Autodesk Inventor part; units mm, degrees
ref_plane "YZ Plane" through (0, 0, 0) normal (1, 0, 0) x (0, 1, 0)
ref_plane "XZ Plane" through (0, 0, 0) normal (0, 1, 0) x (-1, 0, 0)
ref_plane "XY Plane" through (0, 0, 0) normal (0, 0, 1) x (1, 0, 0)
sketch "Boceto1" plane through (0, 0, 0) normal (0, 0, 1) x (1, 0, 0)
  line L0 (-71.1055, 70.4875) -> (71.7516, 70.4875) construction
  line L1 (71.7516, 70.4875) -> (71.7516, -69.9887) construction
  line L2 (71.7516, -69.9887) -> (-71.1055, -69.9887) construction
  line L3 (-71.1055, -69.9887) -> (-71.1055, 70.4875) construction
  line L4 (-16.344, -18.0372) -> (15.0954, -18.0372)
  point P0 (0, 0)
sketch "Boceto2" plane through (0, 0, 0) normal (0, 0, 1) x (1, 0, 0)
  line L0 (-30.1866, -53.4632) -> (28.6068, -53.4632)
  line L1 (28.6068, -53.4632) -> (28.6068, -45.7841)
  line L2 (28.6068, -45.7841) -> (25.4871, -40.2647)
  line L3 (25.4871, -40.2647) -> (25.4871, -33.3055)
  line L4 (25.4871, -33.3055) -> (19.4878, -25.8663)
  line L5 (19.4878, -25.8663) -> (17.4099, -23.2897)
  line L6 (17.4099, -23.2897) -> (17.4099, -19.147)
  line L7 (17.4099, -19.147) -> (15.8731, -17.2414)
  line L8 (15.8731, -17.2414) -> (15.8731, -13.8176)
  line L9 (15.8731, -13.8176) -> (28.6068, -13.8176)
  line L10 (28.6068, -13.8176) -> (28.6068, 15.1601)
  line L11 (-30.1866, -53.4632) -> (-30.1866, -45.7841)
  line L12 (-30.1866, -45.7841) -> (-26.4512, -40.2647)
  line L13 (-26.4512, -40.2647) -> (-27.2401, -37.2121)
  line L14 (-27.2401, -37.2121) -> (-27.2401, -33.9857)
  line L15 (-27.2401, -33.9857) -> (-19.5651, -22.6451)
  line L16 (-19.5651, -22.6451) -> (-19.5651, -19.9512)
  line L17 (-19.5651, -19.9512) -> (-16.9146, -18.1942)
  line L18 (-16.9146, -18.1942) -> (-16.9146, -13.8176)
  line L19 (-16.9146, -13.8176) -> (-24.4978, -13.8176)
  arc A0 (-6.2899, 13.0619) -> (-24.4978, -13.8176) centre (7.8446, -16.1193) ccw
  arc A1 (-6.2899, 13.0619) -> (-2.4548, 26.1011) centre (-14.9411, 22.69) ccw
  line L20 (-2.4548, 26.1011) -> (-10.0959, 22.69)
  line L21 (-10.0959, 22.69) -> (-13.96, 24.3955)
  line L22 (-13.96, 24.3955) -> (-25.9619, 19.0376)
  arc A2 (-30.1866, 30.1701) -> (-25.9619, 19.0376) centre (-21.015, 27.2828) ccw
  line L23 (-30.1866, 30.1701) -> (-19.0004, 38.444)
  line L24 (-19.0004, 38.444) -> (-15.9019, 45.9592)
  line L25 (-15.9019, 45.9592) -> (-7.7883, 50.5452)
  line L26 (-7.7883, 50.5452) -> (-10.0959, 56.9512)
  arc A3 (2.199, 50.5452) -> (-10.0959, 56.9512) centre (-7.6346, 46.6736) ccw
  arc A4 (28.6068, 20.3485) -> (2.199, 50.5452) centre (-1.5881, 20.5877) ccw
  line L27 (28.6068, 20.3485) -> (28.6068, -13.8176)
  line L28 (-16.9146, -13.8176) -> (15.8731, -13.8176)
  point P0 (0, 0)
extrude "Extrusión1" add sketch "Boceto2" along normal blind 10
sketch "Boceto3" plane through (0, 0, 10) normal (0, 0, 1) x (1, 0, 0)
  line L0 (-16.9146, -13.8176) -> (-16.9146, -18.1942)
  line L1 (15.8731, -17.2414) -> (15.8731, -13.8176)
  line L2 (-16.9146, -13.8176) -> (15.8731, -13.8176)
  line L3 (15.8731, -13.8176) -> (15.8731, -17.2414)
  line L4 (15.8731, -17.2414) -> (17.4099, -21.9355)
  line L5 (17.4099, -23.2897) -> (17.4099, -19.147)
  line L6 (17.4099, -21.9355) -> (17.4099, -23.2897)
  line L7 (17.4099, -23.2897) -> (18.0548, -23.9053)
  line L8 (25.4871, -40.2647) -> (25.4871, -33.3055)
  line L9 (29.7175, -53.186) -> (29.9979, -54.0424)
  line L10 (29.9979, -54.0424) -> (29.9979, -53.186)
  line L11 (29.9979, -53.186) -> (-30.6163, -53.186)
  line L12 (-30.6163, -53.186) -> (-30.6163, -42.5113)
  line L13 (-30.6163, -42.5113) -> (-26, -41)
  line L14 (-27.2401, -33.9857) -> (-27.2401, -37.2121)
  line L15 (-26, -41) -> (-27.2401, -37.2121)
  line L16 (-27.2401, -37.2121) -> (-27.2401, -33.9857)
  line L17 (-27.2401, -33.9857) -> (-19.7765, -26.1669)
  line L18 (-19.7765, -26.1669) -> (-19.7765, -18.6785)
  line L19 (-19.7765, -18.6785) -> (-15.3627, -17.2335)
  line L20 (-15.3627, -17.2335) -> (-16.9146, -13.8176)
  line L21 (0, 0) -> (-0.3092, -53.186)
  line L22 (29.7175, -53.186) -> (29.7175, -46)
  line L23 (28.6068, -45.7841) -> (25.4871, -40.2647)
  line L24 (29.7175, -46) -> (25.4871, -40.2647)
  line L25 (25.4871, -33.3055) -> (17.4099, -23.2897)
  line L26 (25.4871, -33.3055) -> (17.4099, -23.2897)
  line L27 (-24.4978, -13.8176) -> (-16.9146, -13.8176)
  line L28 (-16.9146, -13.8176) -> (15.8731, -13.8176)
properties part number "KINGHT 1.0"
Input: part model. Units: mm. Frame: model coordinates. A direction names the side the tool comes from. Coordinates: 2 decimals unless noted, no trailing zeros. Loops run counter-clockwise (first coordinate to the right, second up) from the corner with the lowest first, then second, coordinate; pieces in that order, holes last. Notation, with made-up numbers: M 39,55.25 L 88,55.25 A15 cw 88,65.25 Z; hole C -30,75.25 d6. An arc over 180 degrees is marked long. Use a Markdown table: item, result. Add a question column.
1) Section C-C, the plane y = -15. Return the cut outline in (x, z), plus the area to 3 significant figures.
2) Set-up query: faces 1 (the flat face through (-1, 3, 10)), 2 (the flat face through (-19.877, 21.754, 4.93)), 3 (the flat face through (-21, -13.818, 5)), 4 (the flat face through (-1, -53.463, 5)), 5 (the flat face through (17.41, -21, 5)). Return all of +Z, -Z, +X, -X, +Y, -Y with unobstructed straight access to the full face (end or side cutting, diameter ignored); none if empty.
3) Draft query along X for faces 6 (the flat face through (-12, 23.53, 4.93)), 7 (the flat face through (28.607, -50, 5)), 8 (the cylindrical face through (-19.13, 1.87, 4.93)). Return one class per face: +X half, -X half, draft (parallel to the pull), parting line (faces both ways), or undercut.
4) Pin query (flat end, axial travel): P1, Ø2, axis at y = -21.5, z = 3.5, coming from the -X side; P2, Ø6, axis at y = -49, z = 3, coming from the -X side; P3, Ø1.7, axis at y = -16, z = 3.5, coming from the +X side. Return the tip coordinate at first contact, or that it passes through.
5) Section D-D, the plane x = 6. Return the cut outline in (y, z), plus the area to 3 significant figures.
6) Line query: L1, parallel to Y at x = -19, z = 8; L2, parallel to Y at x = 20, z = 9; L3, parallel to Y at x = -25, z = 9. Output: solid intervals per line, ascending. Write a range as from..to.
7) Section B-B, the plane x = -22. Return the cut outline in (y, z).
Answer below:
| question | item | result |
|---|---|---|
| 1 | outline | M -16.91,0 L 15.87,0 L 15.87,10 L -16.91,10 Z |
| 1 | area | 328 mm2 |
| 2 | face 1 | +Z, +X, -X, +Y, -Y |
| 2 | face 2 | +Z, -Z |
| 2 | face 3 | +Z, -Z, -X |
| 2 | face 4 | +Z, -Z, +X, -X, -Y |
| 2 | face 5 | +Z, -Z, +X |
| 3 | face 6 | undercut |
| 3 | face 7 | +X half |
| 3 | face 8 | -X half |
| 4 | P1 | x = -19.57 |
| 4 | P2 | x = -30.19 |
| 4 | P3 | x = 15.87 |
| 5 | outline | M -53.46,0 L 49.81,0 L 49.81,10 L -53.46,10 Z |
| 5 | area | 1,030 mm2 |
| 6 | L1 | -53.46..-19.58, -13.82..2.07, 22.15..38.44 |
| 6 | L2 | -53.46..-26.5, -13.82..41.7 |
| 6 | L3 | -53.46..-30.68, 19.47..34.01 |
| 7 | outline | M -53.46,0 L -26.24,0 L -26.24,10 L -53.46,10 Z; M -13.82,0 L -3.45,0 L -3.45,10 L -13.82,10 Z; M 20.81,0 L 36.23,0 L 36.23,10 L 20.81,10 Z |
